Work out the finished part from the listing and answer in its coordinate system (mm). A direction names the side the tool comes from. Round coordinates to 2 decimals unless told otherwise and drop trailing zeros. Loops run counter-clockwise (first coordinate to the right, second up) from the corner with the lowest first, then second, coordinate; pieces in that order, holes last. Notation, with made-up numbers: (-7.75, 84.5) - (16.25, 84.5) arc R27 cw to (16.25, 103.5) - close; hole circle Ø5 at (53, 19.5). An arc over 180 degrees is marked (long way). Answer as CSV lines item,"result". Start each with the question number.
Q1. Section A-A on x = -4 is taken. Write down the section's boundary in (y, z), then the cut area to 3 significant figures.
Q2. For faces 5 (the face through (-112, 110, 30.5)), 6 (the face through (-81, 142.5, 35)), 7 (the face through (-25, 99, -1)), determine the directions among +Z, -Z, +X, -X, +Y, -Y from which every point of the face is accessible in a straight line to the end or side of a thin tool.
Q3. Section C-C on x = -80 is taken. Write down the section's boundary in (y, z), then the cut area to 3 significant figures.
Q4. Section D-D on y = 184 is taken. Write down the section's boundary in (x, z).
Q5. Section B-B on y = 100 is taken. Write down the section's boundary in (x, z), then the cut area to 3 significant figures.
Q6. Each of these flat-tipped pins is pushed along its axis until it touches: pin 1 Ø10 at (y, z) = (44, -43.5) entering from -X; pin 2 Ø8 at (x, z) = (-86.5, 36.5) entering from -Y; pin 3 Ø8 at (x, y) = (-11, 116) entering from +Z; pin 4 Ø8 at (x, z) = (-35.5, 22.5) entering from -Y. Where does it stop, or does it pass through?
Q7. The mould has two halves that part along X. Classify faces 1 (the face through (-127.5, 99, -74)), 2 (the face through (-84.231, 132.223, 35.43)), 3 (the face through (-112, 110, -69.5)), 4 (the face through (2.5, 99, 75)): +X half, -X half, draft (parallel to the pull), parting line (faces both ways), or undercut.
Q8. Straight lines are drawn through the part: L1, parallel to Y at x = -80, z = 32.75; L2, parallel to Z at x = -51.5, y = 119; L3, parallel to X at y = 13.5, z = 124. For each, find the intervals that lie inside material, in ascending order. Write a range as [from, to].
```python
from build123d import *

# Parameters (mm, degrees)
F0_W     = 8
F0_H     = 90
F1_DEPTH = 200
F3_W     = 95
F3_H     = 85
F3_R     = 32.5
F4_DEPTH = 10
F6_W     = 95
F6_H     = 85
F6_R     = 32.5
F7_DEPTH = 10


with BuildPart() as f1:
    # F0 (on Front) → F1 (new body)
    with BuildSketch(Plane.XZ):
        with BuildLine():
            Line((2.5, 69.5), (2.5, 80))
            Line((2.5, 80), (-24.5, 80))
            Line((-24.5, 80), (-32.5, 80))
            Line((-32.5, 80), (-32.5, -80))
            Line((-32.5, -80), (32.5, -80))
            Line((32.5, -80), (32.5, -69.5))
            Line((32.5, -69.5), (-19, -69.5))
            ThreePointArc((-19, -69.5), (-23.2426406871, -67.7426406871), (-25, -63.5))
            Line((-25, -63.5), (-25, 63.5))
            ThreePointArc((-25, 63.5), (-23.2426406871, 67.7426406871), (-19, 69.5))
            Line((-19, 69.5), (2.5, 69.5))
        make_face()
        with Locations((-28.5, 125)):
            Rectangle(F0_W, F0_H)
    extrude(amount=-F1_DEPTH)

    # F3 (on offset) → F4 (join)
    with BuildSketch(Plane.XY.offset(-69.5)):
        with Locations((-80, 100)):
            Rectangle(F3_W, F3_H)
        with Locations((-80, 100)):
            Circle(F3_R, mode=Mode.SUBTRACT)
    extrude(amount=-F4_DEPTH)

    # F6 (on offset) → F7 (join)
    with BuildSketch(Plane.XY.offset(30.5)):
        with Locations((-80, 100)):
            Rectangle(F6_W, F6_H)
        with Locations((-80, 100)):
            Circle(F6_R, mode=Mode.SUBTRACT)
    extrude(amount=F7_DEPTH)


solid = f1.part
```
Findings:
1,outline,"(0, -80) - (200, -80) - (200, -69.5) - (0, -69.5) - close; (0, 69.5) - (200, 69.5) - (200, 80) - (0, 80) - close"
1,area,"4,200 mm^2"
2,face 5,"-X, +Y, -Y"
2,face 6,"+Z, -Z, -X, +Y"
2,face 7,"+X, +Y, -Y"
3,outline,"(57.5, -79.5) - (67.5, -79.5) - (67.5, -69.5) - (57.5, -69.5) - close; (57.5, 30.5) - (67.5, 30.5) - (67.5, 40.5) - (57.5, 40.5) - close; (132.5, -79.5) - (142.5, -79.5) - (142.5, -69.5) - (132.5, -69.5) - close; (132.5, 30.5) - (142.5, 30.5) - (142.5, 40.5) - (132.5, 40.5) - close"
3,area,"400 mm^2"
4,outline,"(-32.5, -80) - (32.5, -80) - (32.5, -69.5) - (-19, -69.5) arc R6 cw to (-25, -63.5) - (-25, 63.5) arc R6 cw to (-19, 69.5) - (2.5, 69.5) - (2.5, 80) - (-24.5, 80) - (-24.5, 170) - (-32.5, 170) - close"
5,outline,"(-127.5, -79.5) - (-112.5, -79.5) - (-112.5, -69.5) - (-127.5, -69.5) - close; (-127.5, 30.5) - (-112.5, 30.5) - (-112.5, 40.5) - (-127.5, 40.5) - close; (-47.5, -79.5) - (-32.5, -79.5) - (-32.5, -80) - (32.5, -80) - (32.5, -69.5) - (-19, -69.5) arc R6 cw to (-25, -63.5) - (-25, 63.5) arc R6 cw to (-19, 69.5) - (2.5, 69.5) - (2.5, 80) - (-24.5, 80) - (-24.5, 170) - (-32.5, 170) - (-32.5, 40.5) - (-47.5, 40.5) - (-47.5, 30.5) - (-32.5, 30.5) - (-32.5, -69.5) - (-47.5, -69.5) - close"
5,area,"3,430 mm^2"
6,pin 1,"stops at x = -32.5"
6,pin 2,"stops at y = 57.5"
6,pin 3,"stops at z = 80"
6,pin 4,"stops at y = 0"
7,face 1,"-X half"
7,face 2,"undercut"
7,face 3,"draft"
7,face 4,"+X half"
8,L1,"y = [57.5, 67.5], [132.5, 142.5]"
8,L2,"z = [-79.5, -69.5], [30.5, 40.5]"
8,L3,"x = [-32.5, -24.5]"
